CAD build for the part. Positions are in the model's coordinates, mm. Face numbers are marked on the shaded views. A direction names the side the tool comes from. Give positions to 0.01 mm unless a question says otherwise; leave off trailing zeros. Order: outer loops, then holes, each group sorted by start corner. A loop starts at its lowest first (then second) coordinate and runs counter-clockwise, first axis right, second up.
Item 1: Band-saw the part on D-D on y = 12.5. Give the cut face in (x, z).
Item 2: Band-saw the part on B-B on y = 28. Give the cut face in (x, z), plus the area to 4 significant figures.
Item 3: Band-saw the part on A-A on x = -0.5. Give the cut face in (y, z).
Item 4: Which spindle directions (+Z, -Z, +X, -X, +Y, -Y) get a long thin tool onto all of the face, cutting with end or side? Do the marked faces 4 and 5. Say none if no direction does.
Item 5: Flat gauge pins, fed straight in: P1, Ø2, axis at x = -8, z = -37.5, coming from the +Y side; P2, Ø6, axis at x = 6.5, z = -15, coming from the +Y side; P3, Ø8, axis at x = -12, y = 23.5, coming from the +Z side. Where does each tip first touch, or does it go through?
Item 6: Wall check: L1, parallel to Y at x = -11, z = -44; L2, parallel to Z at x = -1, y = 26; L3, parallel to Y at x = 17.5, z = -9.5. Give the ranges that are in metal, low to high.
Item 7: Two-plate mould, pull along X, no slides. Class the marked faces 1, 2 and 3: released by +X, released by -X, zero draft, split by the parting line, or undercut.
Item 8: Band-saw the part on C-C on z = -30. Give the cut face in (x, y), plus the area to 3 significant figures.
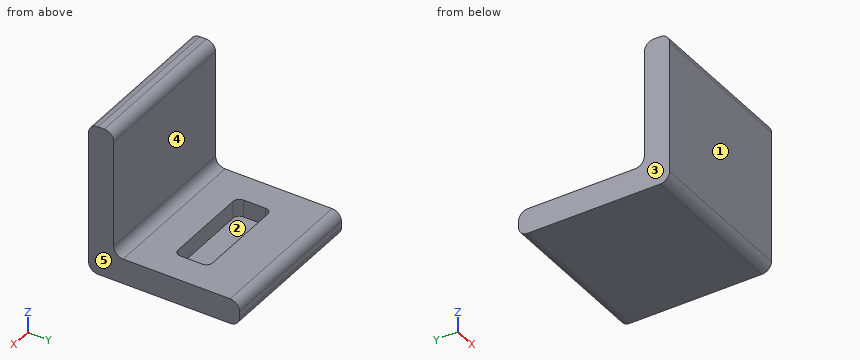
```python
from build123d import *

# Parameters (mm, degrees)
SKETCH1_W           = 50
SKETCH1_H           = 40
BOSS_EXTRUDE1_DEPTH = 8
SKETCH2_W           = 50
SKETCH2_H           = 48
BOSS_EXTRUDE2_DEPTH = 8
SKETCH3_W           = 31
SKETCH3_H           = 11
CUT_EXTRUDE1_DEPTH  = 5.5
FILLET1_R           = 2
FILLET2_R           = 3


with BuildPart() as part:
    # Sketch1 → Boss-Extrude1 (new body)
    with BuildSketch(Plane(origin=(0, 0, 0), x_dir=(1, 0, 0), z_dir=(0, 1, 0))):
        with Locations((0, 20)):
            Rectangle(SKETCH1_W, SKETCH1_H)
    extrude(amount=BOSS_EXTRUDE1_DEPTH)

    # Sketch2 → Boss-Extrude2 (add)
    with BuildSketch(Plane(origin=(0, 0, -40), x_dir=(-1, 0, 0), z_dir=(0, 0, -1))):
        with Locations((0, 24)):
            Rectangle(SKETCH2_W, SKETCH2_H)
    extrude(amount=BOSS_EXTRUDE2_DEPTH)

    # Sketch3 → Cut-Extrude1 (cut)
    with BuildSketch(Plane.XY.offset(-40)):
        with Locations((0, 26.5)):
            Rectangle(SKETCH3_W, SKETCH3_H)
    extrude(amount=-CUT_EXTRUDE1_DEPTH, mode=Mode.SUBTRACT)

    # Fillet1
    fillet1_edges = [part.edges().sort_by_distance(p)[0] for p in [
        (-15.5, 21, -42.75),
        (-15.5, 32, -42.75),
        (15.5, 32, -42.75),
        (15.5, 21, -42.75),
    ]]
    fillet(fillet1_edges, radius=FILLET1_R)

    # Fillet2
    fillet2_edges = [part.edges().sort_by_distance(p)[0] for p in [
        (0, 48, -40),
        (0, 0, -48),
        (0, 8, -40),
        (0, 48, -48),
        (0, 0, 0),
        (0, 8, 0),
    ]]
    fillet(fillet2_edges, radius=FILLET2_R)


solid = part.part
```
The answers:
1. outline: (-25, -48) - (25, -48) - (25, -40) - (-25, -40) - close
2. outline: (-25, -48) - (25, -48) - (25, -40) - (15.5, -40) - (15.5, -45.5) - (-15.5, -45.5) - (-15.5, -40) - (-25, -40) - close
2. area: 229.5 mm2
3. outline: (0, -45) arc R3 ccw to (3, -48) - (45, -48) arc R3 ccw to (48, -45) - (48, -43) arc R3 ccw to (45, -40) - (32, -40) - (32, -45.5) - (21, -45.5) - (21, -40) - (11, -40) arc R3 cw to (8, -37) - (8, -3) arc R3 ccw to (5, 0) - (3, 0) arc R3 ccw to (0, -3) - close
4. face 4: +Z, +X, -X, +Y
4. face 5: +Z, -Z, +X, +Y, -Y
5. P1: stops at y = 8.4
5. P2: stops at y = 8
5. P3: stops at z = -40
6. L1: y = 0 to 21, 32 to 48
6. L2: z = -48 to -45.5
6. L3: y = 0 to 8
7. face 1: zero draft
7. face 2: undercut
7. face 3: released by -X
8. outline: (-25, 0) - (25, 0) - (25, 8) - (-25, 8) - close
8. area: 400 mm2
